Part print with two shaded views. Sizes in mm from the minimum x, y, z corner. Round coordinates to 2 decimals unless told otherwise and drop trailing zeros. Order: outer loops, then holes, each group sorted by start corner. A loop starts at its lowest first (then second) coordinate and runs counter-clockwise, first axis right, second up. Notation, with made-up numbers: (-34.75, 38) -> (-29.75, 38) arc R35 ccw to (-29.75, 73) -> close; hole circle Ø1 at (66.5, 82.25). An arc over 180 degrees is marked (long way). Use a Markdown table: item, result. Add a question column.
Item 1: Probe L1, parallel to X at y = 0.65, z = 48.45 (3 decimals); L2, parallel to Z at x = 12.5, y = 2.7; L3, parallel to Z at x = 12, y = 0.85. List the from-to ranges inside material, lowest first.
Item 2: Slice it at A-A, the plane z = 48. Give the cut face in (x, y), plus the area to 3 significant figures.
Item 3: Two-plate mould, pull along Y, no slides. Class the marked faces 1 and 2: released by +Y, released by -Y, zero draft, split by the parting line, or undercut.
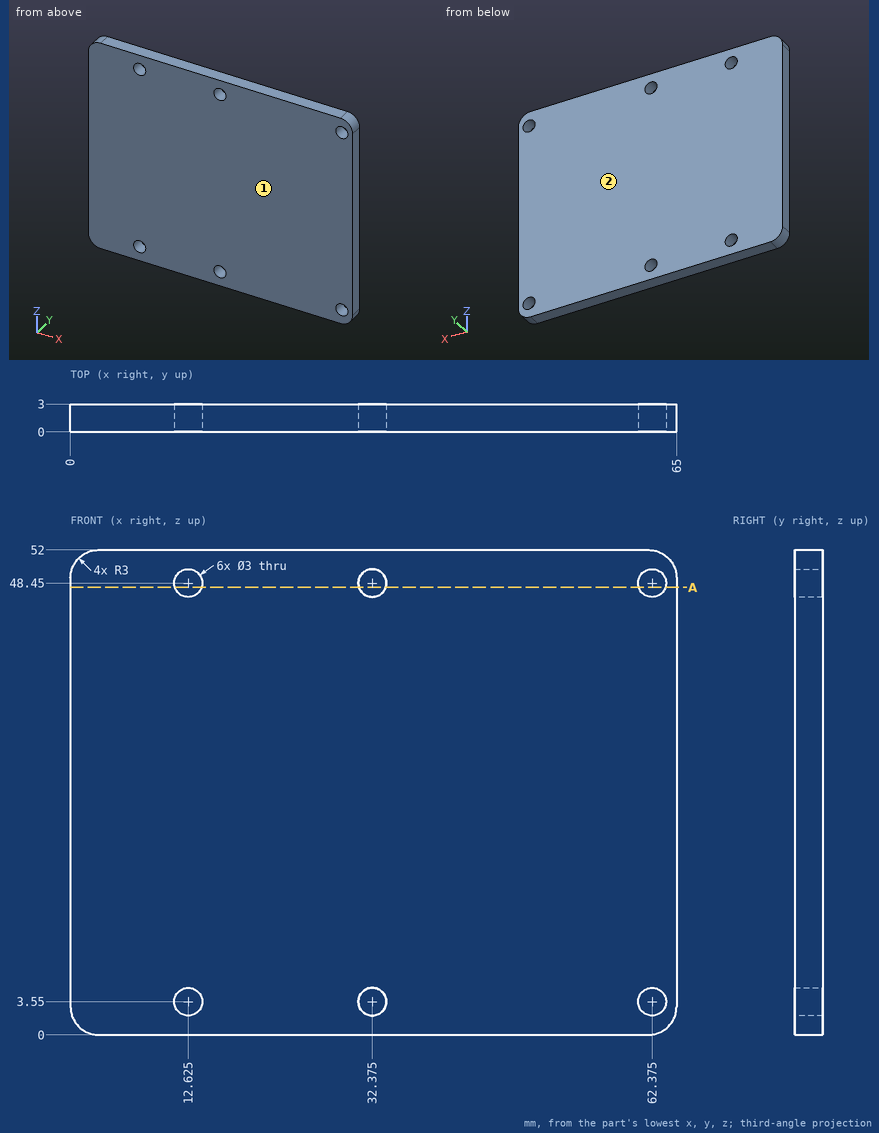
Check sheet entries:
| question | item | result |
|---|---|---|
| 1 | L1 | 0 to 11.125, 14.125 to 30.875, 33.875 to 60.875, 63.875 to 65 |
| 1 | L2 | 0 to 2.06, 5.04 to 46.96, 49.94 to 52 |
| 1 | L3 | 0 to 2.19, 4.91 to 47.09, 49.81 to 52 |
| 2 | outline | (0, 0) -> (11.19, 0) -> (11.19, 3) -> (0, 3) -> close; (14.06, 0) -> (30.94, 0) -> (30.94, 3) -> (14.06, 3) -> close; (33.81, 0) -> (60.94, 0) -> (60.94, 3) -> (33.81, 3) -> close; (63.81, 0) -> (65, 0) -> (65, 3) -> (63.81, 3) -> close |
| 2 | area | 169 mm2 |
| 3 | face 1 | released by -Y |
| 3 | face 2 | released by +Y |
